For this review, take the finished solid that the model builds, in its own axes (mm). A direction names the side the tool comes from. Coordinates: 2 decimals unless noted, no trailing zeros. Write each loop counter-clockwise with the first axis right and the second up, starting at its lowest first coordinate (ties: lowest second). Pieces come first, ordered by that corner, then holes.
```python
from build123d import *

# Parameters (mm, degrees)
F1_DEPTH = 152.4
F2_W     = 254
F2_H     = 38.1
F3_DEPTH = 88.9


with BuildPart() as f1:
    # F0 (on Front) → F1 (new body)
    with BuildSketch(Plane.XZ):
        Polygon((812.8, 101.6), (-812.8, 101.6), (-850.9, -101.6), (850.9, -101.6), align=None)
    extrude(amount=F1_DEPTH)

    # F2 (on face) → F3 (cut)
    with BuildSketch(Plane(origin=(0, 0, -101.6), x_dir=(1, 0, 0), z_dir=(0, 0, -1))):
        with Locations((-723.9, 73.66)):
            Rectangle(F2_W, F2_H)
        with Locations((723.9, 76.2)):
            Rectangle(F2_W, F2_H)
    extrude(amount=-F3_DEPTH, mode=Mode.SUBTRACT)


solid = f1.part
```
Q1. Add section B-B (z = -77.5). State the section outline as (x, y) points, then the cut area to 3 significant figures.
Ans:
outline: (-846.38, -152.4) - (846.38, -152.4) - (846.38, -95.25) - (596.9, -95.25) - (596.9, -57.15) - (846.38, -57.15) - (846.38, 0) - (-846.38, 0) - (-846.38, -54.61) - (-596.9, -54.61) - (-596.9, -92.71) - (-846.38, -92.71) - close
area: 239,000 mm2
Q2. For probe 1 along Y at (x, z) = (732.5, -19); probe 2 along X at (y, z) = (-69.5, -85.5); probe 3 along Y at (x, z) = (-636, -45.5), list the stretches that pass through material, from the lowest coordinate up.
Ans:
probe 1: y = -152.4 to -95.25, -57.15 to 0
probe 2: x = -596.9 to 596.9
probe 3: y = -152.4 to -92.71, -54.61 to 0
Q3. Add section C-C (y = -122.5). State the section outline as (x, z) points, then the cut area to 3 significant figures.
Ans:
outline: (-850.9, -101.6) - (850.9, -101.6) - (812.8, 101.6) - (-812.8, 101.6) - close
area: 338,000 mm2
Q4. Add section D-D (z = 32). State the section outline as (x, y) points.
Ans:
outline: (-825.85, -152.4) - (825.85, -152.4) - (825.85, 0) - (-825.85, 0) - close
Q5. Draft analysis for pull direction Y (two halves, no side actions). For faces 4 (the flat face through (-12, 0, 1)), 5 (the flat face through (596.9, -76, -58)), 6 (the flat face through (11, -75, 101.6)), state which applies: +Y half, -Y half, draft (parallel to the pull), parting line (faces both ways), or undercut.
Ans:
face 4: +Y half
face 5: undercut
face 6: draft
Q6. Clearance check with flat-ended pins moving along their axes: pin 1 Ø19 at (x, y) = (676.5, -82) entering from -Z; pin 2 Ø19 at (y, z) = (-79.5, -53) entering from +X; pin 3 Ø19 at (y, z) = (-64.5, -44) entering from -X. State where each tip first meets the part, or that it passes through.
Ans:
pin 1: stops at z = -12.7
pin 2: stops at x = 596.9
pin 3: stops at x = -596.9
Q7. Add section A-A (x = 643.5). State the section outline as (y, z) points, then the cut area to 3 significant figures.
Ans:
outline: (-152.4, -101.6) - (-95.25, -101.6) - (-95.25, -12.7) - (-57.15, -12.7) - (-57.15, -101.6) - (0, -101.6) - (0, 101.6) - (-152.4, 101.6) - close
area: 27,600 mm2
Q8. Tool access review of faces 1 (the flat face through (832.117, -75.133, -1.422)), 2 (the flat face through (722, -95.25, -58)), 3 (the flat face through (-596.9, -73, -58)): name each direction out of +Z, -Z, +X, -X, +Y, -Y from which nothing blocks a thin tool from reaching the whole face with its end or side.
Ans:
face 1: +Z, +X, +Y, -Y
face 2: -Z, +X
face 3: -Z, -X
